from build123d import *

# Parameters (mm, degrees)
SKETCH_1_R      = 4
EXTRUDE_1_DEPTH = 4


with BuildPart() as part:
    # 草图1 → 凸台-拉伸1 (new body)
    with BuildSketch(Plane.XY):
        with BuildLine():
            ThreePointArc((3.948047826, 9.187650318), (-5.50088728, 8.351062156), (-10, 0))
            add(Edge.make_bspline(
                [(-10, 0), (-10.890214237, -19.135341361), (75, -21.401956932)],
                knots=[0, 0, 0, 1, 1, 1], degree=2))
            add(Edge.make_bspline(
                [(160, 0), (160.890214237, -19.135341361), (75, -21.401956932)],
                knots=[0, 0, 0, 1, 1, 1], degree=2))
            ThreePointArc((160, 0), (155.415713455, 8.40654791), (145.865990446, 9.105490926))
            add(Edge.make_bspline(
                [(3.948047826, 9.187650318), (46.906488456, -20.373746255), (110.551742639, -16.70704022), (145.865990446, 9.105490926)],
                knots=[0.022448948, 0.022448948, 0.022448948, 0.022448948, 0.850781246, 0.850781246, 0.850781246, 0.850781246], degree=3))
        make_face()
        Circle(SKETCH_1_R, mode=Mode.SUBTRACT)
        with Locations((150, 0)):
            Circle(SKETCH_1_R, mode=Mode.SUBTRACT)
    extrude(amount=EXTRUDE_1_DEPTH)


solid = part.part
Geometry check sheet. Reference: the model listing, model coordinates, mm. Give positions to 0.01 mm unless a question says otherwise; leave off trailing zeros.
1) Gauge pin test, flat end, axial feed: pin 1 (1.5 mm diameter, centred on x = 127, z = 1.5, fed in from -Y). Record the tip position at first contact, or that the pin passes through.
Results are:
pin 1: stops at y = -17.48
2) Draft check along X on faces 1 (the flat face through (74, -12, 4)), 2 (the cylindrical face through (-5.38, 8.43, 1.97)). Enter one of: released by +X, released by -X, zero draft, split by the parting line, or undercut.
Results are:
face 1: zero draft
face 2: undercut
3) Cross-section at A-A (z = 1.3). Give the number of separate pieces and of enclosed holes in the cut face, then the cut area to 3 significant figures.
Results are:
separate pieces: 1
enclosed holes: 2
area: 2,310 mm2
4) Material ranges on probe 1 along X at (y, z) = (5.5, 2.25); probe 2 along Y at (x, z) = (149, 3.45); probe 3 along Y at (x, z) = (150, 2.05), recorded low to high.
Results are:
probe 1: x = -8.35 to 9.7, 140.52 to 158.35
probe 2: y = -11.76 to -3.87, 3.87 to 9.95
probe 3: y = -11.32 to -4, 4 to 10
